Can you work these out from the model? Positions are in its coordinate system, mm. Round coordinates to 2 decimals unless told otherwise and drop trailing zeros. Write each loop counter-clockwise with the first axis right and the second up, starting at its lowest first coordinate (ties: lowest second). Pieces come first, ordered by that corner, then holes. Notation, with made-up numbers: (11.25, 44.25) -> (40.25, 44.25) arc R20 ccw to (40.25, 53.25) -> close; hole circle Ø1 at (18.25, 42.5). An arc over 180 degrees is marked (long way). Write item = value, one per line. Start each with the question number.
1) Imagine slicing it at A-A, the plane z = -16. Please give me the cut outline in (x, y).
2) Imagine slicing it at C-C, the plane x = -55. Please give me the cut outline in (y, z), then the cut area to 3 significant figures.
3) If I drill on line 1 (X direction, y = 4.25, z = -17); line 2 (Z direction, x = -55, y = 2.5); line 3 (X direction, y = 2.5, z = 15), over which ranges is the centre line in solid material (lowest first)?
4) Thinking about a two-plate mould opening in Z: for faces 1 (the face through (51.88, 3.22, 14.08)), 2 (the face through (73.19, 3.22, 28.9)), 3 (the face through (-76.2, 3, 0)), which applies, +Z half, -Z half, draft (parallel to the pull), parting line (faces both ways), or undercut?
5) Imagine slicing it at B-B, the plane y = 1.25. Please give me the cut outline in (x, z).
6) Imagine slicing it at D-D, the plane x = 0. Please give me the cut outline in (y, z), then the cut area to 3 significant figures.
from build123d import *

# Parameters (mm, degrees)
SKETCH1_W           = 152.4
SKETCH1_H           = 63.5
BOSS_EXTRUDE1_DEPTH = 6.35
FILLET1_R           = 10
CUT_EXTRUDE4_DEPTH  = 6.35
SKETCH2_R           = 5
CUT_EXTRUDE5_DEPTH  = 10


with BuildPart() as part:
    # Sketch1 → Boss-Extrude1 (new body)
    with BuildSketch(Plane(origin=(0, 0, 0), x_dir=(1, 0, 0), z_dir=(0, 1, 0))):
        Rectangle(SKETCH1_W, SKETCH1_H)
    extrude(amount=BOSS_EXTRUDE1_DEPTH)

    # Fillet1
    fillet1_edges = [part.edges().sort_by_distance(p)[0] for p in [
        (76.2, 3.175, 31.75),
        (-76.2, 3.175, 31.75),
        (-76.2, 3.175, -31.75),
        (76.2, 3.175, -31.75),
    ]]
    fillet(fillet1_edges, radius=FILLET1_R)

    # Sketch3 → Cut-Extrude4 (cut)
    with BuildSketch(Plane(origin=(0, 6.35, 0), x_dir=(1, 0, 0), z_dir=(0, 1, 0))):
        with BuildLine():
            Line((-12.7, 31.75), (12.7, 31.75))
            ThreePointArc((12.7, 31.75), (0, 19.05), (-12.7, 31.75))
        make_face()
    extrude(amount=-CUT_EXTRUDE4_DEPTH, mode=Mode.SUBTRACT)

    # Sketch2 → Cut-Extrude5 (cut)
    with BuildSketch(Plane(origin=(0, 6.35, 0), x_dir=(1, 0, 0), z_dir=(0, 1, 0))):
        with Locations((-55.5625, 17.4625)):
            Circle(SKETCH2_R)
        with Locations((55.5625, 17.4625)):
            Circle(SKETCH2_R)
        with Locations((55.5625, -17.4625)):
            Circle(SKETCH2_R)
        with Locations((-55.5625, -17.4625)):
            Circle(SKETCH2_R)
    extrude(amount=-CUT_EXTRUDE5_DEPTH, mode=Mode.SUBTRACT)


solid = part.part
Reported:
q1.outline = (-76.2, 0) -> (-60.34, 0) -> (-60.34, 6.35) -> (-76.2, 6.35) -> close; (-50.78, 0) -> (50.78, 0) -> (50.78, 6.35) -> (-50.78, 6.35) -> close; (60.34, 0) -> (76.2, 0) -> (76.2, 6.35) -> (60.34, 6.35) -> close
q2.outline = (0, -31.75) -> (6.35, -31.75) -> (6.35, -22.43) -> (0, -22.43) -> close; (0, -12.49) -> (6.35, -12.49) -> (6.35, 12.49) -> (0, 12.49) -> close; (0, 22.43) -> (6.35, 22.43) -> (6.35, 31.75) -> (0, 31.75) -> close
q2.area = 277 mm²
q3.line_1 = -76.2 to -60.54, -50.58 to 50.58, 60.54 to 76.2
q3.line_2 = -31.75 to -22.43, -12.49 to 12.49, 22.43 to 31.75
q3.line_3 = -76.2 to -59.91, -51.21 to 51.21, 59.91 to 76.2
q4.face_1 = undercut
q4.face_2 = +Z half
q4.face_3 = draft
q5.outline = (-76.2, -21.75) arc R10 ccw to (-66.2, -31.75) -> (-12.7, -31.75) arc R12.7 cw to (12.7, -31.75) -> (66.2, -31.75) arc R10 ccw to (76.2, -21.75) -> (76.2, 21.75) arc R10 ccw to (66.2, 31.75) -> (-66.2, 31.75) arc R10 ccw to (-76.2, 21.75) -> close; hole circle Ø10 at (-55.56, -17.46); hole circle Ø10 at (-55.56, 17.46); hole circle Ø10 at (55.56, -17.46); hole circle Ø10 at (55.56, 17.46)
q6.outline = (0, -19.05) -> (6.35, -19.05) -> (6.35, 31.75) -> (0, 31.75) -> close
q6.area = 323 mm²
